Part model, mm, in its own coordinate system. Face numbers are marked on the shaded views. A direction names the side the tool comes from. Round coordinates to 2 decimals unless told otherwise and drop trailing zeros. Order: outer loops, then holes, each group sorted by start corner. A loop starts at its lowest first (then second) coordinate and runs counter-clockwise, first axis right, second up. Notation, with made-up numbers: (44, 42.5) -> (53, 42.5) arc R26 cw to (53, 60.5) -> close; hole circle Ø2 at (45.5, -1). An arc over 180 degrees is marked (long way). Use CSV: the item, a comma, the result in double quotes.
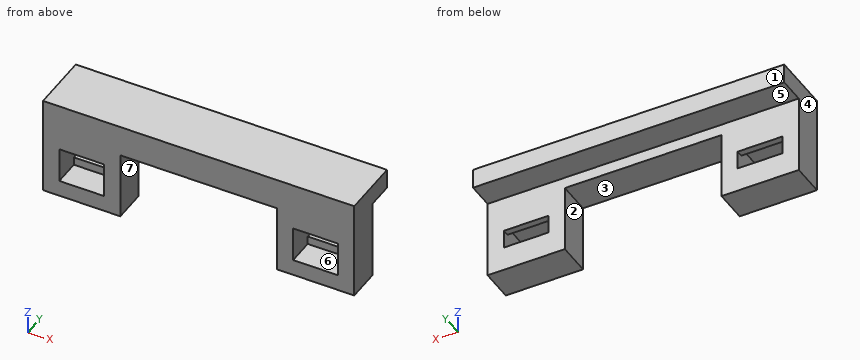
```python
from build123d import *

# Parameters (mm, degrees)
SKETCH1_W           = 59.944
SKETCH1_H           = 19.05
SKETCH1_W_2         = 8.636
SKETCH1_H_2         = 6.7564
BOSS_EXTRUDE1_DEPTH = 5.08
SKETCH2_W           = 59.944
SKETCH2_H           = 19.05
SKETCH2_W_2         = 8.636
SKETCH2_H_2         = 3.5814
BOSS_EXTRUDE2_DEPTH = 1.27
SKETCH5_W           = 30.1625
SKETCH5_H           = 13.0302
CUT_EXTRUDE1_DEPTH  = 30.48
SKETCH6_W           = 59.944
SKETCH6_H           = 3.81
BOSS_EXTRUDE4_DEPTH = 5.08


with BuildPart() as part:
    # Sketch1 → Boss-Extrude1 (new body)
    with BuildSketch(Plane(origin=(0, 0, 0), x_dir=(1, 0, 0), z_dir=(0, 1, 0))):
        with Locations((-29.450443736, 19.033631364)):
            Rectangle(SKETCH1_W, SKETCH1_H)
        with Locations((-51.967543736, 22.030831364)):
            Rectangle(SKETCH1_W_2, SKETCH1_H_2, mode=Mode.SUBTRACT)
        with Locations((-6.920643736, 22.030831364)):
            Rectangle(SKETCH1_W_2, SKETCH1_H_2, mode=Mode.SUBTRACT)
    extrude(amount=BOSS_EXTRUDE1_DEPTH)

    # Sketch2 → Boss-Extrude2 (add)
    with BuildSketch(Plane(origin=(0, 5.08, 0), x_dir=(1, 0, 0), z_dir=(0, 1, 0))):
        with Locations((-29.450443736, 19.033631364)):
            Rectangle(SKETCH2_W, SKETCH2_H)
        with Locations((-51.967543736, 22.030831364)):
            Rectangle(SKETCH2_W_2, SKETCH2_H_2, mode=Mode.SUBTRACT)
        with Locations((-6.920643736, 22.030831364)):
            Rectangle(SKETCH2_W_2, SKETCH2_H_2, mode=Mode.SUBTRACT)
    extrude(amount=BOSS_EXTRUDE2_DEPTH)

    # Sketch5 → Cut-Extrude1 (cut)
    with BuildSketch(Plane.XZ):
        with Locations((-29.444093736, -22.043531364)):
            Rectangle(SKETCH5_W, SKETCH5_H)
    extrude(amount=-CUT_EXTRUDE1_DEPTH, mode=Mode.SUBTRACT)

    # Sketch6 → Boss-Extrude4 (add)
    with BuildSketch(Plane(origin=(0, 6.35, 0), x_dir=(1, 0, 0), z_dir=(0, 1, 0))):
        with Locations((-29.450443736, 11.413631364)):
            Rectangle(SKETCH6_W, SKETCH6_H)
    extrude(amount=BOSS_EXTRUDE4_DEPTH)


solid = part.part
```
(1) Cut at A-A, the plane z = -24.5. Give the cut face in (x, y).
Reply:
outline,"(-59.42, 0) -> (-56.29, 0) -> (-56.29, 5.08) -> (-47.65, 5.08) -> (-47.65, 0) -> (-44.53, 0) -> (-44.53, 6.35) -> (-59.42, 6.35) -> close; (-14.36, 0) -> (-11.24, 0) -> (-11.24, 5.08) -> (-2.6, 5.08) -> (-2.6, 0) -> (0.52, 0) -> (0.52, 6.35) -> (-14.36, 6.35) -> close"
(2) Pull direction X, two halves, no side cores. Call the marked faces 1, 2, 3 and 4: released by +X, released by -X, zero draft, split by the parting line, or undercut.
Reply:
face 1,"zero draft"
face 2,"undercut"
face 3,"undercut"
face 4,"released by -X"
(3) Drop flat-ended pins along their axis: P1, Ø0.5, axis at x = -52, z = -19, coming from the -Y side; P2, Ø3, axis at x = -28.5, y = 2.5, coming from the -Z side; P3, Ø1.5, axis at x = -21, y = 9.5, coming from the -Z side; P4, Ø1.3, axis at x = -51.5, z = -25, coming from the -Y side. Give the stop position or say it passes through.
Reply:
P1,"y = 5.08"
P2,"z = -15.53"
P3,"z = -13.32"
P4,"y = 0"
(4) Cut at C-C, the plane y = 1. Give the cut face in (x, z).
Reply:
outline,"(-59.42, -28.56) -> (-44.53, -28.56) -> (-44.53, -15.53) -> (-14.36, -15.53) -> (-14.36, -28.56) -> (0.52, -28.56) -> (0.52, -9.51) -> (-59.42, -9.51) -> close; hole (-56.29, -25.41) -> (-47.65, -25.41) -> (-47.65, -18.65) -> (-56.29, -18.65) -> close; hole (-11.24, -25.41) -> (-2.6, -25.41) -> (-2.6, -18.65) -> (-11.24, -18.65) -> close"
(5) Which spindle directions (+Z, -Z, +X, -X, +Y, -Y) get a long thin tool onto all of the face, cutting with end or side? Do the marked faces 5, 6 and 7. Say none if no direction does.
Reply:
face 5,"-Z, +X, -X, +Y"
face 6,"-Y"
face 7,"-Z, +Y, -Y"
(6) Cut at D-D, the plane x = -12.5. Give the cut face in (y, z).
Reply:
outline,"(0, -28.56) -> (6.35, -28.56) -> (6.35, -13.32) -> (11.43, -13.32) -> (11.43, -9.51) -> (0, -9.51) -> close"
(7) Cut at B-B, the plane x = -52.5. Give the cut face in (y, z).
Reply:
outline,"(0, -28.56) -> (6.35, -28.56) -> (6.35, -23.82) -> (5.08, -23.82) -> (5.08, -25.41) -> (0, -25.41) -> close; (0, -18.65) -> (5.08, -18.65) -> (5.08, -20.24) -> (6.35, -20.24) -> (6.35, -13.32) -> (11.43, -13.32) -> (11.43, -9.51) -> (0, -9.51) -> close"
(8) Probe probe 1 along X at (y, z) = (3.25, -24.75); probe 2 along X at (y, z) = (3, -26.5); probe 3 along Z at (x, y) = (-4.5, 1.25). List the from-to ranges inside material, lowest first. Write a range as [from, to].
Reply:
probe 1,"[-59.42, -56.29], [-47.65, -44.53], [-14.36, -11.24], [-2.6, 0.52]"
probe 2,"[-59.42, -44.53], [-14.36, 0.52]"
probe 3,"[-28.56, -25.41], [-18.65, -9.51]"
